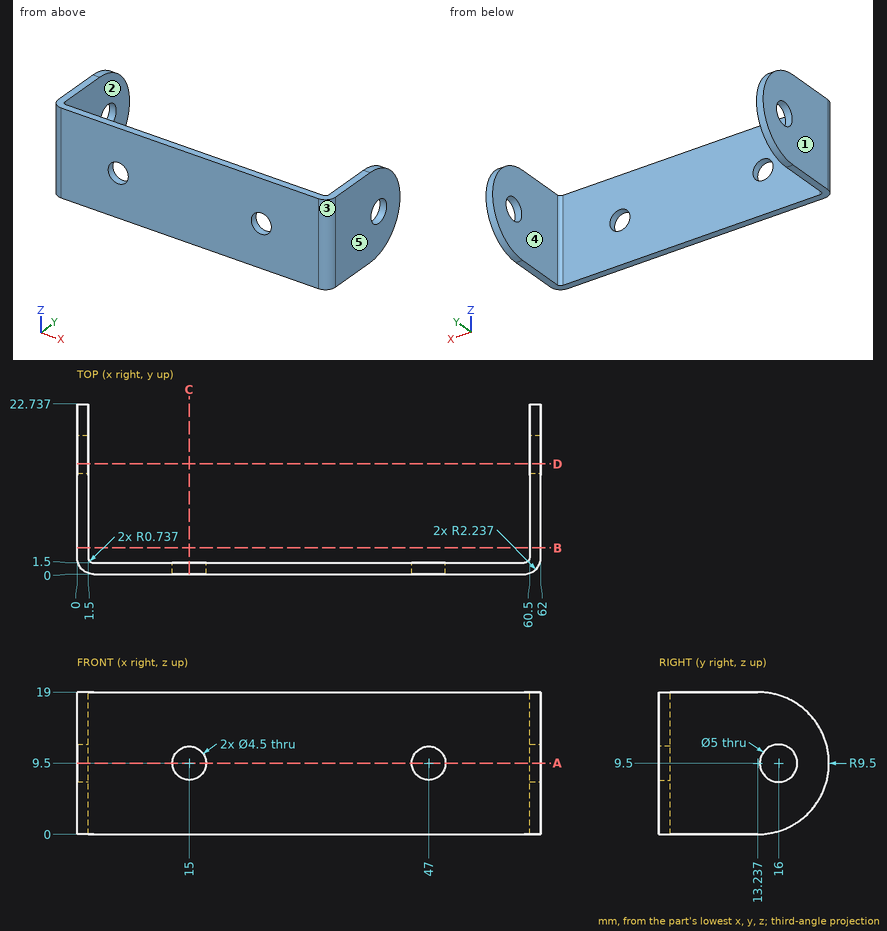
The drawing under review shows one solid part. Ordinate dimensions are in mm from its lowest x, y, z. A direction names the side the tool comes from. Round coordinates to 2 decimals unless told otherwise and drop trailing zeros. Order: outer loops, then holes, each group sorted by start corner. A loop starts at its lowest first (then second) coordinate and runs counter-clockwise, first axis right, second up. Notation, with made-up numbers: (32, -35) -> (75, -35) arc R15 cw to (75, -15) -> close; hole circle Ø4 at (73.5, 30.5). An arc over 180 degrees is marked (long way). Return JSON: item names as keys, results as strings.
1. Take a section at B-B (y = 3.5). Write out the cut boundary in (x, z).
Answer block:
{"outline": "(0, 0) -> (1.5, 0) -> (1.5, 19) -> (0, 19) -> close; (60.5, 0) -> (62, 0) -> (62, 19) -> (60.5, 19) -> close"}
2. For the marked faces 4 and 5, list the 3-axis set-ups (+Z, -Z, +X, -X, +Y, -Y) from which the entire face can be reached by the end or side of a thin tool; tool diameter is ignored.
Answer block:
{"face 4": "+Z, -Z, +Y", "face 5": "+Z, -Z, +X, +Y, -Y"}
3. Insertion check: P1, Ø1.5, axis at x = 25, z = 15.5, coming from the +Y side; P2, Ø4.5, axis at y = 16, z = 9.5, coming from the +X side. Each pin has a flat end and moves straight along its axis. Give the tip position at first contact, or say it passes through.
Answer block:
{"P1": "stops at y = 1.5", "P2": "passes through"}
4. Take a section at C-C (x = 15). Write out the cut boundary in (y, z).
Answer block:
{"outline": "(0, 0) -> (1.5, 0) -> (1.5, 7.25) -> (0, 7.25) -> close; (0, 11.75) -> (1.5, 11.75) -> (1.5, 19) -> (0, 19) -> close"}
5. The part is to be moulded in two halves that separate along X. For the marked faces 1, 2 and 3, say which applies: +X half, -X half, draft (parallel to the pull), parting line (faces both ways), or undercut.
Answer block:
{"face 1": "-X half", "face 2": "undercut", "face 3": "+X half"}
6. Take a section at D-D (y = 14.75). Write out the cut boundary in (x, z) (1 decimal).
Answer block:
{"outline": "(0, 0.1) -> (1.5, 0.1) -> (1.5, 7.3) -> (0, 7.3) -> close; (0, 11.7) -> (1.5, 11.7) -> (1.5, 18.9) -> (0, 18.9) -> close; (60.5, 0.1) -> (62, 0.1) -> (62, 7.3) -> (60.5, 7.3) -> close; (60.5, 11.7) -> (62, 11.7) -> (62, 18.9) -> (60.5, 18.9) -> close"}
7. For L1, parallel to X at y = 8.25, z = 13.5; L2, parallel to Y at x = 39.5, z = 15; L3, parallel to Z at x = 61.3, y = 16, list the stretches that pass through material, from the lowest coordinate up. Write a range as [from, to].
Answer block:
{"L1": "x = [0, 1.5], [60.5, 62]", "L2": "y = [0, 1.5]", "L3": "z = [0.41, 7], [12, 18.59]"}
8. Take a section at A-A (z = 9.5). Write out the cut boundary in (x, y).
Answer block:
{"outline": "(0, 2.24) arc R2.24 ccw to (2.24, 0) -> (12.75, 0) -> (12.75, 1.5) -> (2.24, 1.5) arc R0.74 cw to (1.5, 2.24) -> (1.5, 13.5) -> (0, 13.5) -> close; (0, 18.5) -> (1.5, 18.5) -> (1.5, 22.74) -> (0, 22.74) -> close; (17.25, 0) -> (44.75, 0) -> (44.75, 1.5) -> (17.25, 1.5) -> close; (49.25, 0) -> (59.76, 0) arc R2.24 ccw to (62, 2.24) -> (62, 13.5) -> (60.5, 13.5) -> (60.5, 2.24) arc R0.74 cw to (59.76, 1.5) -> (49.25, 1.5) -> close; (60.5, 18.5) -> (62, 18.5) -> (62, 22.74) -> (60.5, 22.74) -> close"}
